Source: CAD feature listing. Evaluate the final solid. Frame: model axes, mm. Give positions to 0.01 mm unless a question says otherwise; leave off trailing zeros. Order: outer loops, then holes, each group sorted by start corner. A loop starts at its lowest first (then second) coordinate and runs counter-clockwise, first axis right, second up. Notation, with made-up numbers: (52, 19.25) - (102, 19.25) arc R14 cw to (102, 46.25) - close; hole circle Ø3 at (-31, 29). An arc over 180 degrees is marked (long way). Answer as CSV lines item,"result".
```python
from build123d import *

# Parameters (mm, degrees)
BASEPLATE_OUTLINE_R = 2.1
BASEPLATE_DEPTH     = 2.8
CUT_EXTRUDE1_REACH  = 115.438
SKETCH3_W           = 15.4
SKETCH3_H           = 19.3
SKETCH3_W_2         = 15.6
SKETCH3_W_3         = 16.2
SKETCH3_H_2         = 24.9
SKETCH3_W_4         = 3.7
SKETCH3_H_3         = 2.4
CUT_EXTRUDE2_REACH  = 115.438
SKETCH4_W           = 6.9
SKETCH4_H           = 5.4


# Read off the part's stored shape, not the designer's step: BasePlate
with BuildPart() as part:
    # BasePlate outline → BasePlate (new body)
    with BuildSketch(Plane(origin=(0, 0, 0), x_dir=(1, 0, 0), z_dir=(0, 1, 0))):
        with BuildLine():
            Line((43.502626614, -5.852332608), (48.792614178, -5.852332608))
            ThreePointArc((48.792614178, -5.852332608), (49.082078508, -5.760021707), (49.264659986, -5.517174213))
            Line((49.264659986, -5.517174213), (50.078201202, -3.187491002))
            ThreePointArc((50.078201202, -3.187491002), (50.26078268, -2.944643509), (50.55024701, -2.852332608))
            Line((50.55024701, -2.852332608), (58.116695703, -2.852332608))
            ThreePointArc((58.116695703, -2.852332608), (58.484685739, -3.013831008), (58.614956567, -3.393999275))
            ThreePointArc((58.614956567, -3.393999275), (64.799237397, -7.61016844), (65.229166667, -0.137781095))
            ThreePointArc((65.229166667, -0.137781095), (65.061014427, 0.043158816), (65, 0.282515593))
            Line((65, 0.282515593), (65, 83.012819192))
            ThreePointArc((65, 83.012819192), (65.061014427, 83.252175969), (65.229166667, 83.433115879))
            ThreePointArc((65.229166667, 83.433115879), (65.940559159, 90.088226551), (59.285448487, 89.376834059))
            ThreePointArc((59.285448487, 89.376834059), (59.104508577, 89.208681819), (58.8651518, 89.147667392))
            Line((58.8651518, 89.147667392), (6.1348482, 89.147667392))
            ThreePointArc((6.1348482, 89.147667392), (5.895491423, 89.208681819), (5.714551513, 89.376834059))
            ThreePointArc((5.714551513, 89.376834059), (-0.940559159, 90.088226551), (-0.229166667, 83.433115879))
            ThreePointArc((-0.229166667, 83.433115879), (-0.061014427, 83.252175969), (0, 83.012819192))
            Line((0, 83.012819192), (0, 0.282515593))
            ThreePointArc((0, 0.282515593), (-0.061014427, 0.043158816), (-0.229166667, -0.137781095))
            ThreePointArc((-0.229166667, -0.137781095), (0.200762603, -7.61016844), (6.385043433, -3.393999275))
            ThreePointArc((6.385043433, -3.393999275), (6.515314261, -3.013831008), (6.883304297, -2.852332608))
            Line((6.883304297, -2.852332608), (14.44975299, -2.852332608))
            ThreePointArc((14.44975299, -2.852332608), (14.73921732, -2.944643509), (14.921798798, -3.187491002))
            Line((14.921798798, -3.187491002), (15.735340014, -5.517174213))
            ThreePointArc((15.735340014, -5.517174213), (15.917921492, -5.760021707), (16.207385822, -5.852332608))
            Line((16.207385822, -5.852332608), (21.497373386, -5.852332608))
            ThreePointArc((21.497373386, -5.852332608), (21.786837716, -5.760021707), (21.969419194, -5.517174213))
            Line((21.969419194, -5.517174213), (22.78296041, -3.187491002))
            ThreePointArc((22.78296041, -3.187491002), (22.965541888, -2.944643509), (23.255006218, -2.852332608))
            Line((23.255006218, -2.852332608), (41.744993782, -2.852332608))
            ThreePointArc((41.744993782, -2.852332608), (42.034458112, -2.944643509), (42.21703959, -3.187491002))
            Line((42.21703959, -3.187491002), (43.030580806, -5.517174213))
            ThreePointArc((43.030580806, -5.517174213), (43.213162284, -5.760021707), (43.502626614, -5.852332608))
        make_face()
        with Locations((2.1, -3.752332608)):
            Circle(BASEPLATE_OUTLINE_R, mode=Mode.SUBTRACT)
        with Locations((62.9, -3.752332608)):
            Circle(BASEPLATE_OUTLINE_R, mode=Mode.SUBTRACT)
        with Locations((2.1, 87.047667392)):
            Circle(BASEPLATE_OUTLINE_R, mode=Mode.SUBTRACT)
        with Locations((62.9, 87.047667392)):
            Circle(BASEPLATE_OUTLINE_R, mode=Mode.SUBTRACT)
    extrude(amount=BASEPLATE_DEPTH)

    # Sketch3 → Cut-Extrude1 (cut, up to next)
    with BuildSketch(Plane(origin=(0, 2.8, 0), x_dir=(1, 0, 0), z_dir=(0, 1, 0)), mode=Mode.PRIVATE) as cut_extrude1_sk1:
        Polygon((9, 0.647667392), (54.7, 0.647667392), (54.7, 6.647667392), (63, 6.647667392), (63, 4.147667392), (65, 4.147667392), (65, 42.047667392), (63, 42.047667392), (63, 40.047667392), (35.4, 40.047667392), (35.4, 61.647667392), (31.8, 61.647667392), (31.8, 66.147667392), (15.8, 66.147667392), (15.8, 61.647667392), (4.7, 61.647667392), (4.7, 2.647667392), (9, 2.647667392), align=None)
    cut_extrude1_tool1 = extrude(cut_extrude1_sk1.sketch, amount=-CUT_EXTRUDE1_REACH, mode=Mode.PRIVATE) & part.part
    # Sketch3 → Cut-Extrude1 (cut, up to next)
    with BuildSketch(Plane(origin=(0, 2.8, 0), x_dir=(1, 0, 0), z_dir=(0, 1, 0)), mode=Mode.PRIVATE) as cut_extrude1_sk2:
        with Locations((14, 79.497667392)):
            Rectangle(SKETCH3_W, SKETCH3_H)
    cut_extrude1_tool2 = extrude(cut_extrude1_sk2.sketch, amount=-CUT_EXTRUDE1_REACH, mode=Mode.PRIVATE) & part.part
    # Sketch3 → Cut-Extrude1 (cut, up to next)
    with BuildSketch(Plane(origin=(0, 2.8, 0), x_dir=(1, 0, 0), z_dir=(0, 1, 0)), mode=Mode.PRIVATE) as cut_extrude1_sk3:
        with Locations((32, 79.497667392)):
            Rectangle(SKETCH3_W_2, SKETCH3_H)
    cut_extrude1_tool3 = extrude(cut_extrude1_sk3.sketch, amount=-CUT_EXTRUDE1_REACH, mode=Mode.PRIVATE) & part.part
    # Sketch3 → Cut-Extrude1 (cut, up to next)
    with BuildSketch(Plane(origin=(0, 2.8, 0), x_dir=(1, 0, 0), z_dir=(0, 1, 0)), mode=Mode.PRIVATE) as cut_extrude1_sk4:
        with Locations((51, 76.697667392)):
            Rectangle(SKETCH3_W_3, SKETCH3_H_2)
    cut_extrude1_tool4 = extrude(cut_extrude1_sk4.sketch, amount=-CUT_EXTRUDE1_REACH, mode=Mode.PRIVATE) & part.part
    # Sketch3 → Cut-Extrude1 (cut, up to next)
    with BuildSketch(Plane(origin=(0, 2.8, 0), x_dir=(1, 0, 0), z_dir=(0, 1, 0)), mode=Mode.PRIVATE) as cut_extrude1_sk5:
        with Locations((11.35, 66.847667392)):
            Rectangle(SKETCH3_W_4, SKETCH3_H_3)
    cut_extrude1_tool5 = extrude(cut_extrude1_sk5.sketch, amount=-CUT_EXTRUDE1_REACH, mode=Mode.PRIVATE) & part.part
    add(cut_extrude1_tool1.solids().sort_by_distance((31.029219, 2.8, -28.401895))[0], mode=Mode.SUBTRACT)
    add(cut_extrude1_tool2.solids().sort_by_distance((14, 2.8, -79.497667))[0], mode=Mode.SUBTRACT)
    add(cut_extrude1_tool3.solids().sort_by_distance((32, 2.8, -79.497667))[0], mode=Mode.SUBTRACT)
    add(cut_extrude1_tool4.solids().sort_by_distance((51, 2.8, -76.697667))[0], mode=Mode.SUBTRACT)
    add(cut_extrude1_tool5.solids().sort_by_distance((11.35, 2.8, -66.847667))[0], mode=Mode.SUBTRACT)

    # Sketch4 → Cut-Extrude2 (cut, up to next)
    with BuildSketch(Plane(origin=(0, 2.8, 0), x_dir=(1, 0, 0), z_dir=(0, 1, 0)), mode=Mode.PRIVATE) as cut_extrude2_sk1:
        Polygon((65, 59.347667392), (63, 59.347667392), (63, 57.347667392), (54.4, 57.347667392), (54.4, 61.747667392), (51.9, 61.747667392), (51.9, 59.847667392), (42.4, 59.847667392), (42.4, 57.947667392), (40.05, 57.947667392), (40.05, 47.947667392), (38.2, 47.947667392), (38.2, 42.447667392), (60.9, 42.447667392), (60.9, 50.047667392), (63, 50.047667392), (63, 48.047667392), (65, 48.047667392), align=None)
    cut_extrude2_tool1 = extrude(cut_extrude2_sk1.sketch, amount=-CUT_EXTRUDE2_REACH, mode=Mode.PRIVATE) & part.part
    # Sketch4 → Cut-Extrude2 (cut, up to next)
    with BuildSketch(Plane(origin=(0, 2.8, 0), x_dir=(1, 0, 0), z_dir=(0, 1, 0)), mode=Mode.PRIVATE) as cut_extrude2_sk2:
        with Locations((36.95, 65.647667392)):
            Rectangle(SKETCH4_W, SKETCH4_H)
    cut_extrude2_tool2 = extrude(cut_extrude2_sk2.sketch, amount=-CUT_EXTRUDE2_REACH, mode=Mode.PRIVATE) & part.part
    add(cut_extrude2_tool1.solids().sort_by_distance((51.243501, 2.8, -50.961182))[0], mode=Mode.SUBTRACT)
    add(cut_extrude2_tool2.solids().sort_by_distance((36.95, 2.8, -65.647667))[0], mode=Mode.SUBTRACT)


solid = part.part
```
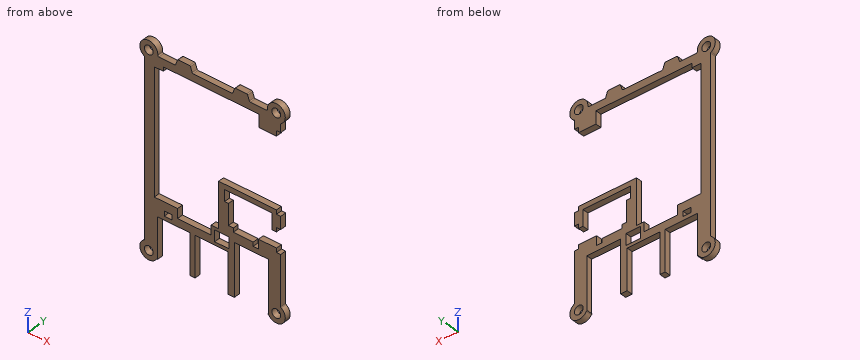
(1) Cut plane B-B (x = 2.1). Return loops of the section in (y, z).
Completed:
outline,"(0, -91.35) - (2.8, -91.35) - (2.8, -89.15) - (0, -89.15) - close; (0, -84.95) - (2.8, -84.95) - (2.8, 1.65) - (0, 1.65) - close; (0, 5.85) - (2.8, 5.85) - (2.8, 8.05) - (0, 8.05) - close"
(2) Ray query, line 1 (Z direction, x = 2.1, y = 1.95); line 2 (Z direction, x = 62.9, y = 1.5); line 3 (X direction, y = 0.4, z = -83). Return the intervals inside material, ascending. Write a range as from..to.
Completed:
line 1,"-91.35..-89.15, -84.95..1.65, 5.85..8.05"
line 2,"-91.35..-89.15, -84.95..-57.35, -50.05..-40.05, -6.65..1.65, 5.85..8.05"
line 3,"0..6.3, 21.7..24.2, 39.8..42.9, 59.1..65"
(3) Cut plane C-C (z = -30). Return loops of the section in (x, y), then the cut area to 3 significant figures.
Completed:
outline,"(0, 0) - (4.7, 0) - (4.7, 2.8) - (0, 2.8) - close"
area,"13.2 mm²"
(4) Contact query for flat-ended pins moving along their axis: pin 1 (0.8 mm diameter, centred on x = 36.5, y = 1.5, fed in from +Z); pin 2 (1.4 mm diameter, centred on x = 14, y = 2, fed in from -Z); pin 3 (0.8 mm diameter, centred on y = 1.5, z = -6, fed in from +X). Output: stop coordinate, or through.
Completed:
pin 1,"z = 2.85"
pin 2,"z = -69.85"
pin 3,"x = 63"
(5) Cut plane D-D (y = 2.05). Give the number of separate pieces and of enclosed holes in the cut face, then the cut area to 3 significant figures.
Completed:
separate pieces,"1"
enclosed holes,"6"
area,"1,600 mm²"
(6) Cut plane A-A (x = 45). Return loops of the section in (y, z), then the cut area to 3 significant figures.
Completed:
outline,"(0, -64.25) - (2.8, -64.25) - (2.8, -59.85) - (0, -59.85) - close; (0, -42.45) - (2.8, -42.45) - (2.8, -40.05) - (0, -40.05) - close; (0, -0.65) - (2.8, -0.65) - (2.8, 5.85) - (0, 5.85) - close"
area,"37.2 mm²"
